Build history of the part. All positions in model axes, mm. Coordinates: 2 decimals unless noted, no trailing zeros. Loops run counter-clockwise (first coordinate to the right, second up) from the corner with the lowest first, then second, coordinate; pieces in that order, holes last. Notation, with made-up numbers: (80.25, 36) - (90.25, 36) arc R30 cw to (90.25, 60) - close; hole circle Ø1 at (88.5, -34). An arc over 180 degrees is marked (long way). One line per item, written item: value.
```python
from build123d import *

# Parameters (mm, degrees)
SKETCH3_W               = 139.7
SKETCH3_H               = 76.2
BOSS_EXTRUDE1_DEPTH     = 3.175
SKETCH4_W               = 119.38
SKETCH4_H               = 38.1
BOSS_EXTRUDE2_DEPTH     = 3.302
SKETCH6_W               = 129.54
SKETCH6_H               = 38.1
BOSS_EXTRUDE3_DEPTH     = 2.54
SKETCH7_W               = 129.54
SKETCH7_H               = 9.017
BOSS_EXTRUDE4_DEPTH     = 2.54
CUT_EXTRUDE1_DEPTH      = 160.237743528
CUT_EXTRUDE1_DEPTH_BACK = 160.237743528
SKETCH8_R               = 3.175


with BuildPart() as part:
    # Sketch3 → Boss-Extrude1 (new body)
    with BuildSketch(Plane.XY):
        with Locations((69.85, -38.1)):
            Rectangle(SKETCH3_W, SKETCH3_H)
    extrude(amount=BOSS_EXTRUDE1_DEPTH)

    # Sketch4 → Boss-Extrude2 (add)
    with BuildSketch(Plane.XY.offset(3.175)):
        with Locations((69.85, -57.15)):
            Rectangle(SKETCH4_W, SKETCH4_H)
    extrude(amount=BOSS_EXTRUDE2_DEPTH)

    # Sketch6 → Boss-Extrude3 (add)
    with BuildSketch(Plane.XY.offset(6.477)):
        with Locations((69.85, -57.15)):
            Rectangle(SKETCH6_W, SKETCH6_H)
    extrude(amount=BOSS_EXTRUDE3_DEPTH)

    # Sketch7 → Boss-Extrude4 (add)
    with BuildSketch(Plane.XZ.offset(76.2)):
        with Locations((69.85, 4.5085)):
            Rectangle(SKETCH7_W, SKETCH7_H)
    extrude(amount=-BOSS_EXTRUDE4_DEPTH)

    # Sketch8 → Cut-Extrude1 (cut, two sides: drawn at the far end of the back side and taken through both)
    with BuildSketch(Plane.XY.offset(3.175).offset(-CUT_EXTRUDE1_DEPTH_BACK)):
        with Locations((19.05, -12.7)):
            Circle(SKETCH8_R)
        with Locations((69.85, -25.4)):
            Circle(SKETCH8_R)
        with Locations((120.65, -12.7)):
            Circle(SKETCH8_R)
    extrude(amount=CUT_EXTRUDE1_DEPTH + CUT_EXTRUDE1_DEPTH_BACK, mode=Mode.SUBTRACT)


solid = part.part
```
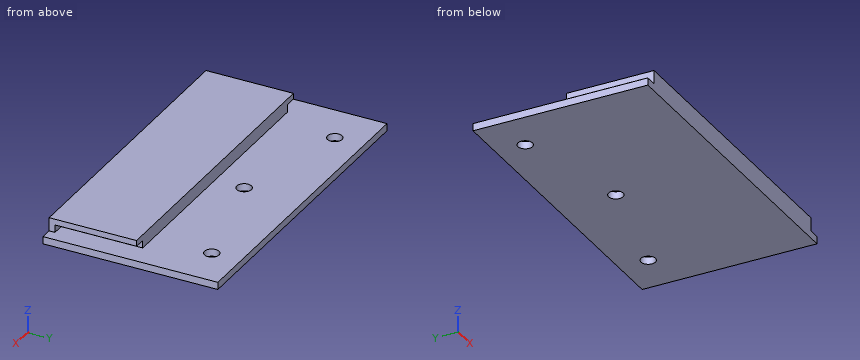
Item 1: Cut at B-B, the plane y = -12.7. Write the cut outline in (x, z) (3 decimals).
Check result:
outline: (0, 0) - (15.875, 0) - (15.875, 3.175) - (0, 3.175) - close; (22.225, 0) - (117.475, 0) - (117.475, 3.175) - (22.225, 3.175) - close; (123.825, 0) - (139.7, 0) - (139.7, 3.175) - (123.825, 3.175) - close
Item 2: Probe probe 1 along X at (y, z) = (-12.7, 1.15) (3 decimals); probe 2 along Y at (x, z) = (120.65, 2.15) (3 decimals); probe 3 along X at (y, z) = (-25.4, 1.5) (3 decimals). List the from-to ranges inside material, lowest first. Write a range as from..to.
Check result:
probe 1: x = 0..15.875, 22.225..117.475, 123.825..139.7
probe 2: y = -76.2..-15.875, -9.525..0
probe 3: x = 0..66.675, 73.025..139.7
Item 3: Drop flat-ended pins along their axis: P1, Ø1.8, axis at x = 86.5, z = 5, coming from the +Y side; P2, Ø1.5, axis at x = 115.5, y = -14, coming from the +Z side (3 decimals); P3, Ø1, axis at y = -55, z = 5, coming from the +X side. Give the stop position or say it passes through.
Check result:
P1: stops at y = -38.1
P2: stops at z = 3.175
P3: stops at x = 129.54
Item 4: Cut at A-A, the plane x = 69.85. Write the cut outline in (y, z) (3 decimals).
Check result:
outline: (-76.2, 0) - (-28.575, 0) - (-28.575, 3.175) - (-38.1, 3.175) - (-38.1, 9.017) - (-76.2, 9.017) - close; (-22.225, 0) - (0, 0) - (0, 3.175) - (-22.225, 3.175) - close
Item 5: Cut at D-D, the plane x = 92. Write the cut outline in (y, z) (3 decimals), then the cut area to 3 significant figures.
Check result:
outline: (-76.2, 0) - (0, 0) - (0, 3.175) - (-38.1, 3.175) - (-38.1, 9.017) - (-76.2, 9.017) - close
area: 465 mm^2
Item 6: Cut at C-C, the plane y = -70. Write the cut outline in (x, z) (3 decimals), then the cut area to 3 significant figures.
Check result:
outline: (0, 0) - (139.7, 0) - (139.7, 3.175) - (129.54, 3.175) - (129.54, 6.477) - (134.62, 6.477) - (134.62, 9.017) - (5.08, 9.017) - (5.08, 6.477) - (10.16, 6.477) - (10.16, 3.175) - (0, 3.175) - close
area: 1,170 mm^2
